```python
from build123d import *

# Parameters (mm, degrees)
SKETCH1_R           = 65
BOSS_EXTRUDE1_DEPTH = 10
SKETCH2_R           = 55
CUT_EXTRUDE1_DEPTH  = 11
SKETCH3_W           = 10
SKETCH3_H           = 5
CUT_EXTRUDE4_DEPTH  = 11


with BuildPart() as part:
    # Sketch1 → Boss-Extrude1 (new body)
    with BuildSketch(Plane.XY):
        Circle(SKETCH1_R)
    extrude(amount=BOSS_EXTRUDE1_DEPTH)

    # Sketch2 → Cut-Extrude1 (cut, through all)
    with BuildSketch(Plane.XY.offset(10)):
        Circle(SKETCH2_R)
    extrude(amount=-CUT_EXTRUDE1_DEPTH, mode=Mode.SUBTRACT)

    # Sketch3 → Cut-Extrude4 (cut, through all)
    with BuildSketch(Plane.XY.offset(10)):
        Polygon((49.461524227, 34.330127019), (53.791651246, 36.830127019), (58.791651246, 28.169872981), (54.461524227, 25.669872981), align=None)
        with Locations((0, 62.5)):
            Rectangle(SKETCH3_W, SKETCH3_H)
        Polygon((54.461524227, -25.669872981), (58.791651246, -28.169872981), (53.791651246, -36.830127019), (49.461524227, -34.330127019), align=None)
        with Locations((0, -62.5)):
            Rectangle(SKETCH3_W, SKETCH3_H)
        Polygon((-49.461524227, -34.330127019), (-53.791651246, -36.830127019), (-58.791651246, -28.169872981), (-54.461524227, -25.669872981), align=None)
        Polygon((-54.461524227, 25.669872981), (-58.791651246, 28.169872981), (-53.791651246, 36.830127019), (-49.461524227, 34.330127019), align=None)
    extrude(amount=-CUT_EXTRUDE4_DEPTH, mode=Mode.SUBTRACT)


solid = part.part
```
Geometry check sheet. Reference: the model listing, model coordinates, mm. A direction names the side the tool comes from. Round coordinates to 2 decimals unless told otherwise and drop trailing zeros. Order: outer loops, then holes, each group sorted by start corner. A loop starts at its lowest first (then second) coordinate and runs counter-clockwise, first axis right, second up. Notation, with made-up numbers: (3, -26.5) -> (50, -26.5) arc R13 ccw to (50, -9.5) -> close; hole circle Ø4 at (27, -14.5). An arc over 180 degrees is marked (long way). Return JSON: item names as keys, results as strings. Group by question number.
Q1. Section check A-A, the plane x = 0. Record the boundary of the cut face in (y, z).
Q2. Section check C-C, the plane z = 7.75. Record the boundary of the cut face in (x, y), plus the area to 3 significant figures.
Q3. Tool access check on faces 4 (the flat face through (0, -60, 5)), 5 (the flat face through (-51.572, 35.549, 5.07)), 6 (the flat face through (51.514, 35.515, 5.07)). Record the directions out of +Z, -Z, +X, -X, +Y, -Y that give a thin tool (end or side, any length) a straight path to the whole face; none if there is none.
Q4. Gauge pin test, flat ends, axial feed: pin 1 (5.5 mm diameter, centred on y = -62.5, z = 2.5, fed in from -X); pin 2 (3 mm diameter, centred on x = 2, z = 5, fed in from -Y); pin 3 (3 mm diameter, centred on x = -2.5, z = 5, fed in from +Y). Record the tip position at first contact, or that the pin passes through.
Q5. Release check for a two-part mould opening along Y. For faces 1 (the flat face through (51.997, 29.939, 5.07)), 2 (the flat face through (56.572, 26.889, 5.07)), 3 (the flat face through (-5, -62, 5)) record: released by +Y, released by -Y, zero draft, split by the parting line, or undercut.
Q6. Material ranges on probe 1 along Y at (x, z) = (0, 7.5); probe 2 along X at (y, z) = (-28, 0.75); probe 3 along Y at (x, z) = (27, 6.5), recorded low to high. Write a range as from..to.
Q7. Section check D-D, the plane x = 51. Record the boundary of the cut face in (y, z), plus the area to 3 significant figures.
Q8. Section check B-B, the plane y = 0. Record the boundary of the cut face in (x, z).
Numbers:
{
 "1": {"outline": "(-60, 0) -> (-55, 0) -> (-55, 10) -> (-60, 10) -> close; (55, 0) -> (60, 0) -> (60, 10) -> (55, 10) -> close"},
 "2": {"outline": "(-58.62, -28.07) -> (-54.46, -25.67) -> (-49.46, -34.33) -> (-53.62, -36.73) arc R65 ccw to (-5, -64.81) -> (-5, -60) -> (5, -60) -> (5, -64.81) arc R65 ccw to (53.62, -36.73) -> (49.46, -34.33) -> (54.46, -25.67) -> (58.62, -28.07) arc R65 ccw to (58.62, 28.07) -> (54.46, 25.67) -> (49.46, 34.33) -> (53.62, 36.73) arc R65 ccw to (5, 64.81) -> (5, 60) -> (-5, 60) -> (-5, 64.81) arc R65 ccw to (-53.62, 36.73) -> (-49.46, 34.33) -> (-54.46, 25.67) -> (-58.62, 28.07) arc R65 ccw to start; hole circle Ø110 at (0, 0)", "area": "3,470 mm^2"},
 "3": {"face 4": "+Z, -Z, -Y", "face 5": "+Z, -Z, -X", "face 6": "+Z, -Z, +X"},
 "4": {"pin 1": "x = -25.59", "pin 2": "y = -60", "pin 3": "y = 60"},
 "5": {"face 1": "undercut", "face 2": "released by +Y", "face 3": "zero draft"},
 "6": {"probe 1": "-60..-55, 55..60", "probe 2": "-58.66..-58.5, -53.12..-47.34, 47.34..53.12, 58.5..58.66", "probe 3": "-59.13..-47.92, 47.92..59.13"},
 "7": {"outline": "(-40.3, 0) -> (-35.22, 0) -> (-35.22, 10) -> (-40.3, 10) -> close; (-31.67, 0) -> (-20.59, 0) -> (-20.59, 10) -> (-31.67, 10) -> close; (20.59, 0) -> (31.67, 0) -> (31.67, 10) -> (20.59, 10) -> close; (35.22, 0) -> (40.3, 0) -> (40.3, 10) -> (35.22, 10) -> close", "area": "323 mm^2"},
 "8": {"outline": "(-65, 0) -> (-55, 0) -> (-55, 10) -> (-65, 10) -> close; (55, 0) -> (65, 0) -> (65, 10) -> (55, 10) -> close"}
}
